Build history of the part. All positions in model axes, mm. A direction names the side the tool comes from. Give positions to 0.01 mm unless a question says otherwise; leave off trailing zeros. Order: outer loops, then holes, each group sorted by start corner. A loop starts at its lowest first (then second) coordinate and runs counter-clockwise, first axis right, second up. Notation, with made-up numbers: (67.5, 49.25) - (110.5, 49.25) arc R23 ccw to (110.5, 81.25) - close; hole circle Ø9 at (3.5, 68.25). An arc over 180 degrees is marked (long way). Answer in a Markdown table with one row per item.
```python
from build123d import *

# Parameters (mm, degrees)
ESBO_O1_W                  = 200
ESBO_O1_H                  = 60
ESBO_O2_W                  = 30
ESBO_O2_H                  = 30
CORTE_EXTRUS_O1_DEPTH      = 201
CORTE_EXTRUS_O1_DEPTH_BACK = 201


with BuildPart() as part:
    # Esboço1 → Revolução1 (revolve)
    with BuildSketch(Plane.XY):
        with Locations((100, 30)):
            Rectangle(ESBO_O1_W, ESBO_O1_H)
    revolve(axis=Axis((0, 0, 0), (0, 1, 0)))

    # Esboço2 → Corte-extrusão1 (cut, two sides)
    with BuildSketch(Plane(origin=(0, 0, 0), x_dir=(0, 0, -1), z_dir=(1, 0, 0))) as corte_extrus_o1_sk:
        with Locations((0, 15)):
            Rectangle(ESBO_O2_W, ESBO_O2_H)
    extrude(amount=CORTE_EXTRUS_O1_DEPTH, mode=Mode.SUBTRACT)
    extrude(corte_extrus_o1_sk.sketch, amount=-CORTE_EXTRUS_O1_DEPTH_BACK, mode=Mode.SUBTRACT)


solid = part.part
```
1. Two-plate mould, pull along Z, no slides. Class faces 1 (the face through (3, 15, -15)), 2 (the face through (184.75, 30.42, 76.6)), 3 (the face through (3, 0, 86)): +Z half, -Z half, draft (parallel to the pull), parting line (faces both ways), or undercut.
Check result:
| item | result |
|---|---|
| face 1 | undercut |
| face 2 | parting line |
| face 3 | draft |
2. Drop flat-ended pins along their axis: P1, Ø1.5, axis at y = 34, z = 37.5, coming from the -X side; P2, Ø8, axis at y = 53.5, z = -155, coming from the +X side; P3, Ø9, axis at x = 27, y = 15.5, coming from the +Z side. Give the stop position or say it passes through.
Check result:
| item | result |
|---|---|
| P1 | stops at x = -196.59 |
| P2 | stops at x = 131.14 |
| P3 | stops at z = 198.73 |
3. Cut at C-C on z = 0. Write the cut outline in (x, y), and give its area (3 significant figures).
Check result:
| item | result |
|---|---|
| outline | (-200, 30) - (200, 30) - (200, 60) - (-200, 60) - close |
| area | 12,000 mm² |
4. Cut at D-D on y = 47.5. Write the cut outline in (x, z).
Check result:
| item | result |
|---|---|
| outline | circle Ø400 at (0, 0) |
5. Cut at A-A on y = 17.5. Write the cut outline in (x, z), and give its area (3 significant figures).
Check result:
| item | result |
|---|---|
| outline | (-199.44, -15) arc R200 ccw to (199.44, -15) - close; (-199.44, 15) - (199.44, 15) arc R200 ccw to start |
| area | 114,000 mm² |
6. Cut at B-B on x = 54. Write the cut outline in (y, z).
Check result:
| item | result |
|---|---|
| outline | (0, -192.57) - (60, -192.57) - (60, 192.57) - (0, 192.57) - (0, 15) - (30, 15) - (30, -15) - (0, -15) - close |
7. Probe line 1 (Z direction, x = 1, y = 24.5); line 2 (Z direction, x = 5, y = 21); line 3 (Y direction, x = -98.5, z = -13). List the from-to ranges inside material, lowest first.
Check result:
| item | result |
|---|---|
| line 1 | z = -200 to -15, 15 to 200 |
| line 2 | z = -199.94 to -15, 15 to 199.94 |
| line 3 | y = 30 to 60 |
8. Which spindle directions (+Z, -Z, +X, -X, +Y, -Y) get a long thin tool onto all of the face, cutting with end or side? Do faces 4 (the face through (-3, 30, 0)), 5 (the face through (3, 0, -88)). Say none if no direction does.
Check result:
| item | result |
|---|---|
| face 4 | +X, -X, -Y |
| face 5 | +Z, -Z, +X, -X, -Y |
